from build123d import *

# Parameters (mm, degrees)
SKETCH1_R            = 5.44942
BOSS_EXTRUDE1_DEPTH  = 2.3815
M3_CLEARANCE_HOLE1_D = 3.2


with BuildPart() as part:
    # Sketch1 → Boss-Extrude1 (new body, symmetric)
    with BuildSketch(Plane(origin=(0, 0, 0), x_dir=(0, 0, -1), z_dir=(1, 0, 0))):
        with BuildLine():
            Line((0, 9.5), (125.5, 22.5))
            Line((125.5, 22.5), (130.263, 22.5))
            Line((130.263, 22.5), (130.263, -22.5))
            Line((130.263, -22.5), (125.5, -22.5))
            Line((125.5, -22.5), (0, -9.5))
            ThreePointArc((0, -9.5), (-9.5, 0), (0, 9.5))
        make_face()
        Circle(SKETCH1_R, mode=Mode.SUBTRACT)
        with BuildLine():
            Line((17.302023212, 6.21531268), (47.183955708, 9.358046468))
            ThreePointArc((47.183955708, 9.358046468), (48.412205474, 8.959031889), (48.9375, 7.779254036))
            Line((48.9375, 7.779254036), (48.9375, -7.779257299))
            ThreePointArc((48.9375, -7.779257299), (48.412206559, -8.959034175), (47.183958614, -9.358050037))
            Line((47.183958614, -9.358050037), (17.302047548, -6.215374112))
            ThreePointArc((17.302047548, -6.215374112), (11.709307369, -4.1665e-05), (17.302023212, 6.21531268))
        make_face(mode=Mode.SUBTRACT)
        with BuildLine():
            Line((120.5, 15.194881882), (120.5, 7.0875))
            ThreePointArc((120.5, 7.0875), (120.035032015, 5.964967985), (118.9125, 5.5))
            Line((118.9125, 5.5), (99.4625, 5.5))
            ThreePointArc((99.4625, 5.5), (98.339967985, 5.964967985), (97.875, 7.0875))
            Line((97.875, 7.0875), (97.875, 13.180140846))
            ThreePointArc((97.875, 13.180140846), (98.283555786, 14.243271501), (99.298932964, 14.759191851))
            Line((99.298932964, 14.759191851), (118.748932964, 16.773932886))
            ThreePointArc((118.748932964, 16.773932886), (119.975630655, 16.373826096), (120.5, 15.194881882))
        make_face(mode=Mode.SUBTRACT)
        with BuildLine():
            Line((120.5, -15.194881882), (120.5, -7.0875))
            ThreePointArc((120.5, -7.0875), (120.035032015, -5.964967985), (118.9125, -5.5))
            Line((118.9125, -5.5), (99.4625, -5.5))
            ThreePointArc((99.4625, -5.5), (98.339967985, -5.964967985), (97.875, -7.0875))
            Line((97.875, -7.0875), (97.875, -13.180140846))
            ThreePointArc((97.875, -13.180140846), (98.283555786, -14.243271501), (99.298932964, -14.759191851))
            Line((99.298932964, -14.759191851), (118.748932964, -16.773932886))
            ThreePointArc((118.748932964, -16.773932886), (119.975630655, -16.373826096), (120.5, -15.194881882))
        make_face(mode=Mode.SUBTRACT)
        with BuildLine():
            Line((89.73075, 7.0875), (89.73075, 12.007628894))
            ThreePointArc((89.73075, 12.007628894), (89.206380655, 13.186573108), (87.979682964, 13.586679898))
            Line((87.979682964, 13.586679898), (58.505682964, 10.533596233))
            ThreePointArc((58.505682964, 10.533596233), (57.490305786, 10.017675884), (57.08175, 8.954545229))
            Line((57.08175, 8.954545229), (57.08175, 7.0875))
            ThreePointArc((57.08175, 7.0875), (57.546717985, 5.964967985), (58.66925, 5.5))
            Line((58.66925, 5.5), (88.14325, 5.5))
            ThreePointArc((88.14325, 5.5), (89.265782015, 5.964967985), (89.73075, 7.0875))
        make_face(mode=Mode.SUBTRACT)
        with BuildLine():
            Line((89.73075, -7.0875), (89.73075, -12.007628894))
            ThreePointArc((89.73075, -12.007628894), (89.206380655, -13.186573108), (87.979682964, -13.586679898))
            Line((87.979682964, -13.586679898), (58.505682964, -10.533596233))
            ThreePointArc((58.505682964, -10.533596233), (57.490305786, -10.017675884), (57.08175, -8.954545229))
            Line((57.08175, -8.954545229), (57.08175, -7.0875))
            ThreePointArc((57.08175, -7.0875), (57.546717985, -5.964967985), (58.66925, -5.5))
            Line((58.66925, -5.5), (88.14325, -5.5))
            ThreePointArc((88.14325, -5.5), (89.265782015, -5.964967985), (89.73075, -7.0875))
        make_face(mode=Mode.SUBTRACT)
    extrude(amount=BOSS_EXTRUDE1_DEPTH, both=True)

    # M3 Clearance Hole1 (through all)
    with Locations(Plane(origin=(2.3815, 0, 0), x_dir=(0, 0, -1), z_dir=(1, 0, 0))):
        with Locations((127.8815, 11.25), (127.8815, -11.25)):
            Hole(M3_CLEARANCE_HOLE1_D / 2)


solid = part.part
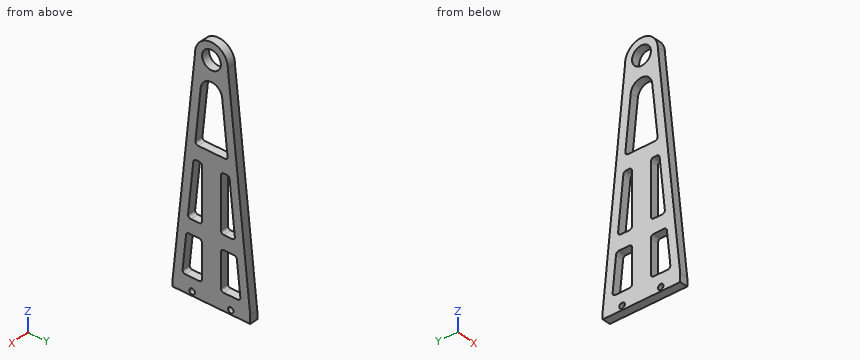
The listing builds one solid part. Answer for the finished solid, in the listing's coordinates (mm). Give positions to 0.01 mm unless a question says otherwise; leave off trailing zeros. Order: outer loops, then holes, each group sorted by start corner. A loop starts at its lowest first (then second) coordinate and runs counter-clockwise, first axis right, second up. Notation, with made-up numbers: (83.25, -4) - (118.25, -4) arc R19 ccw to (118.25, 5) - close; hole circle Ø10 at (32.25, 73.5). An arc over 180 degrees is marked (long way). Use one line per item in the form item = value.
1) Find section C-C on z = -60. Determine the outline of the cut face in (x, y), and give its area (3 significant figures).
Verdict:
outline = (-2.38, -15.72) - (2.38, -15.72) - (2.38, -10.69) - (-2.38, -10.69) - close; (-2.38, -5.5) - (2.38, -5.5) - (2.38, 5.5) - (-2.38, 5.5) - close; (-2.38, 10.69) - (2.38, 10.69) - (2.38, 15.72) - (-2.38, 15.72) - close
area = 100 mm^2
2) Find section A-A on y = 0. Determine the outline of the cut face in (x, z), and give its area (3 significant figures).
Verdict:
outline = (-2.38, -130.26) - (2.38, -130.26) - (2.38, -48.94) - (-2.38, -48.94) - close; (-2.38, -11.71) - (2.38, -11.71) - (2.38, -5.45) - (-2.38, -5.45) - close; (-2.38, 5.45) - (2.38, 5.45) - (2.38, 9.5) - (-2.38, 9.5) - close
area = 436 mm^2
3) Find section D-D on x = 1.6. Give the number of separate pieces and of enclosed holes in the cut face, and give its area (3 significant figures).
Verdict:
separate_pieces = 1
enclosed_holes = 8
area = 2,830 mm^2
4) Consider probe 1 along Z at (x, y) = (-1.8, -0.5); probe 2 along Y at (x, z) = (0.2, -67.5); probe 3 along Y at (x, z) = (1.05, -72). Determine where each line is inside the solid, lowest interval first. Write a range as [from, to].
Verdict:
probe_1 = [-130.26, -48.94], [-11.73, -5.43], [5.43, 9.49]
probe_2 = [-16.49, -11.47], [-5.5, 5.5], [11.47, 16.49]
probe_3 = [-16.96, -11.93], [-5.5, 5.5], [11.93, 16.96]
5) Each of these flat-tipped pins is pushed along its axis until it touches: pin 1 (1.5 mm diameter, centred on x = 0, y = 2.5, fed in from +Z); pin 2 (1.4 mm diameter, centred on x = -1, y = -3, fed in from +Z). Where does it stop, or does it pass through?
Verdict:
pin_1 = 9.34
pin_2 = 9.22
6) Find section B-B on z = -36.5. Determine the outline of the cut face in (x, y), and give its area (3 significant figures).
Verdict:
outline = (-2.38, -13.28) - (2.38, -13.28) - (2.38, -8.23) - (-2.38, -8.23) - close; (-2.38, 8.23) - (2.38, 8.23) - (2.38, 13.28) - (-2.38, 13.28) - close
area = 48.1 mm^2
